Could you check a few things on this model? Use its own coordinates, in mm. A direction names the side the tool comes from. Give positions to 0.01 mm unless a question says otherwise; leave off trailing zeros. Order: outer loops, then holes, each group sorted by start corner. A loop starts at its lowest first (then second) coordinate and runs counter-clockwise, first axis right, second up. Notation, with made-up numbers: (86, 70) -> (97, 70) arc R18 cw to (97, 97) -> close; hole circle Ø2 at (37.25, 46). An arc over 180 degrees is marked (long way). Write each question's results on one line, items separated by ' | '.
```python
from build123d import *

# Parameters (mm, degrees)
F1_DEPTH = 25
F0_W     = 124
F0_H     = 124
F2_DEPTH = 3


with BuildPart() as f1:
    # F0 (on Top) → F1 (new body)
    with BuildSketch(Plane.XY):
        Polygon((47.188934, 11.061991), (-47.153505, 11.061991), (-47.153505, 8.061991), (76.846495, 8.061991), (76.846495, 11.061991), (57.846495, 11.061991), align=None)
        Polygon((-47.153505, 11.061991), (-50.153505, 11.061991), (-50.153505, 9.061991), (-50.153505, -116.938009), (-50.153505, -118.938009), (-47.153505, -118.938009), (-47.153505, -115.938009), (-47.153505, 8.061991), align=None)
        Polygon((76.846495, -115.938009), (-47.153505, -115.938009), (-47.153505, -118.938009), (47.188934, -118.938009), (76.846495, -118.938009), align=None)
        Polygon((76.846495, 11.061991), (76.846495, 8.061991), (76.846495, -115.938009), (76.846495, -118.938009), (79.846495, -118.938009), (79.846495, -116.938009), (79.846495, 11.061991), align=None)
    extrude(amount=F1_DEPTH)

    # F0 (on Top) → F2 (join)
    with BuildSketch(Plane.XY):
        with Locations((14.846495, -53.938009)):
            Rectangle(F0_W, F0_H)
    extrude(amount=F2_DEPTH)


solid = f1.part
```
Q1. Suppose I cut it at A-A on z = 10.75. Please give me the cut outline in (x, y).
Here are the results:
outline: (-50.15, -118.94) -> (79.85, -118.94) -> (79.85, 11.06) -> (-50.15, 11.06) -> close; hole (-47.15, -115.94) -> (76.85, -115.94) -> (76.85, 8.06) -> (-47.15, 8.06) -> close
Q2. Thinking about a two-plate mould opening in Y: for faces 3 (the flat face through (76.846, -53, 14)), 4 (the flat face through (14, -118.938, 12)), 5 (the flat face through (9.7, -116.2, 25)), 6 (the flat face through (14, -53, 3)), which applies, +Y half, -Y half, draft (parallel to the pull), parting line (faces both ways), or undercut?
Here are the results:
face 3: undercut | face 4: -Y half | face 5: draft | face 6: undercut
Q3. For faces 1 (the flat face through (16, 11.062, 12)), 2 (the flat face through (14, 8.062, 14)), which set-ups out of +Z, -Z, +X, -X, +Y, -Y let a thin tool reach every point of the face, with its end or its side?
Here are the results:
face 1: +Z, -Z, +X, -X, +Y | face 2: +Z
Q4. I'm going to push a flat-ended pin straight in: pin 1 Ø10 at (x, y) = (-11.5, -87) entering from +Z. Where does the tip first touch, or does it pass through?
Here are the results:
pin 1: stops at z = 3
Q5. I need wall thicknesses on line 1 along X through (y, z) = (-61.5, 22.5); line 2 along Y through (x, z) = (67, 21.25); line 3 along Z through (x, y) = (53, -109). Which ranges of each line are inside material? Lowest first, please.
Here are the results:
line 1: x = -50.15 to -47.15, 76.85 to 79.85 | line 2: y = -118.94 to -115.94, 8.06 to 11.06 | line 3: z = 0 to 3
Q6. Suppose I cut it at C-C on y = -94. Please give me the cut outline in (x, z).
Here are the results:
outline: (-50.15, 0) -> (79.85, 0) -> (79.85, 25) -> (76.85, 25) -> (76.85, 3) -> (-47.15, 3) -> (-47.15, 25) -> (-50.15, 25) -> close
Q7. Suppose I cut it at B-B on x = -22.5. Please give me the cut outline in (y, z), and give its area (3 significant figures).
Here are the results:
outline: (-118.94, 0) -> (11.06, 0) -> (11.06, 25) -> (8.06, 25) -> (8.06, 3) -> (-115.94, 3) -> (-115.94, 25) -> (-118.94, 25) -> close | area: 522 mm²
